The model under review builds one solid part; all positions refer to its coordinate system, in mm. Face numbers are marked on the shaded views. Give positions to 0.01 mm unless a question says otherwise; leave off trailing zeros. Return JSON: item names as keys, results as strings.
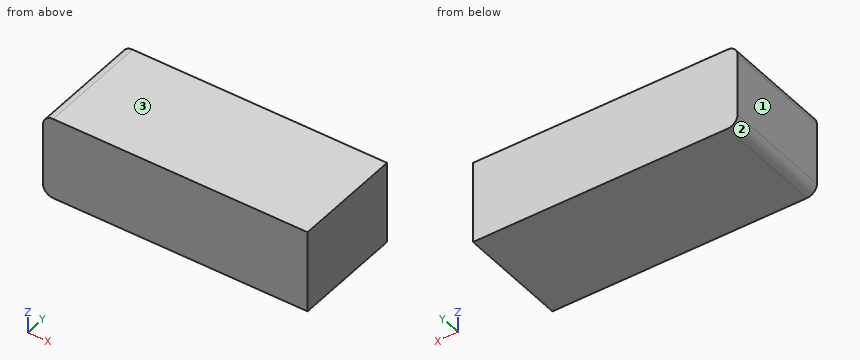
Autodesk Inventor part; units mm, degrees
ref_plane "YZ Plane" through (0, 0, 0) normal (1, 0, 0) x (0, 1, 0)
ref_plane "XZ Plane" through (0, 0, 0) normal (0, 1, 0) x (-1, 0, 0)
ref_plane "XY Plane" through (0, 0, 0) normal (0, 0, 1) x (1, 0, 0)
sketch "Sketch1" plane through (0, 0, 0) normal (0, 0, 1) x (1, 0, 0)
  point P0 (0, 0)
sketch "Sketch2" plane through (0, 0, 0) normal (0, 0, 1) x (1, 0, 0)
  line L0 (-91.5002, 38.5) -> (91.5002, 38.5)
  line L1 (91.5002, 38.5) -> (91.5002, -38.5)
  line L2 (91.5002, -38.5) -> (-91.5002, -38.5)
  line L3 (-91.5002, -38.5) -> (-91.5002, 38.5)
  line L4 (-91.5002, 38.5) -> (91.5002, -38.5) construction
  line L5 (91.5002, 38.5) -> (-91.5002, -38.5) construction
  point P0 (0, 0)
extrude "Extrusion1" add sketch "Sketch2" along normal blind 57
fillet "Fillet1" radius 7 2 edges at (-91.5002, 0, 57) (-91.5002, 0, 0)
properties part number "turnigy_graphene_12Ah"
1) Wall thickness on L1, parallel to X at y = 19.5, z = 54: over which ranges is the line inside the solid? List them lowest first. Write a range as from..to.
From the geometry:
{"L1": "-90.24..91.5"}
2) Insertion check: pin 1 (4 mm diameter, centred on x = -48.5, y = -27, fed in from -Z). The pin has a flat end and moves straight along its axis. Give the tip position at first contact, or say it passes through.
From the geometry:
{"pin 1": "z = 0"}
3) The part is to be moulded in two halves that separate along Z. For the marked faces 1, 2 and 3, say which applies: released by +Z, released by -Z, zero draft, split by the parting line, or undercut.
From the geometry:
{"face 1": "zero draft", "face 2": "released by -Z", "face 3": "released by +Z"}
